Part model, mm, in its own coordinate system. Round coordinates to 2 decimals unless told otherwise and drop trailing zeros. Write each loop counter-clockwise with the first axis right and the second up, starting at its lowest first coordinate (ties: lowest second). Pieces come first, ordered by that corner, then holes. Notation, with made-up numbers: M 54,86 L 99,86 A7 ccw 99,96 Z; hole C 59.25,-21 d1. An arc over 180 degrees is marked long. Use a Markdown table: item, result. Add a question column.
1) Slice it at C-C on z = -3. Write the cut outline in (x, y).
2) Slice it at B-B on x = 20. Write the cut outline in (y, z), plus the area to 3 significant figures.
3) Drop flat-ended pins along their axis: P1, Ø1, axis at x = -9.5, z = -1, coming from the -Y side; P2, Ø5, axis at x = -29.5, z = 3.5, coming from the -Y side; P3, Ø3, axis at x = 31.5, y = 0, coming from the -Z side. Give the stop position or say it passes through.
4) Wall check: probe 1 along Y at (x, z) = (-17, 0); probe 2 along X at (y, z) = (4, -1); probe 3 along X at (y, z) = (1.5, -3.25). Give the ranges that are in metal, low to high.
5) Slice it at A-A on y = 0. Write the cut outline in (x, z).
```python
from build123d import *

# Parameters (mm, degrees)
SKETCH1_R      = 1.27
EXTRUDE1_DEPTH = 44.45


with BuildPart() as part:
    # Sketch1 → Extrude1 (new, symmetric)
    with BuildSketch(Plane(origin=(0, 0, 0), x_dir=(0, 0, -1), z_dir=(1, 0, 0))):
        Circle(SKETCH1_R)
    extrude(amount=EXTRUDE1_DEPTH, both=True)

    # Sketch2 → Revolve1 (revolve)
    with BuildSketch(Plane.ZY.offset(44.45)):
        with BuildLine():
            Line((0, -5.1054), (0, 5.1054))
            ThreePointArc((0, 5.1054), (-5.1054, 0), (0, -5.1054))
        make_face()
    revolve(axis=Axis((-44.45, 8.762723072, 0), (0, -1, 0)))

    # Sketch3 → Revolve2 (revolve)
    with BuildSketch(Plane(origin=(44.45, 0, 0), x_dir=(0, 0, -1), z_dir=(1, 0, 0))):
        with BuildLine():
            Line((0, 5.1054), (0, -5.1054))
            ThreePointArc((0, -5.1054), (5.1054, 0), (0, 5.1054))
        make_face()
    revolve(axis=Axis((44.45, 5.1054, 0), (0, -1, 0)))


solid = part.part
```
Entries:
| question | item | result |
|---|---|---|
| 1 | outline | C -44.45,0 d8.26; C 44.45,0 d8.26 |
| 2 | outline | C 0,0 d2.54 |
| 2 | area | 5.07 mm^2 |
| 3 | P1 | stops at y = -1.17 |
| 3 | P2 | stops at y = -0.78 |
| 3 | P3 | stops at z = -1.27 |
| 4 | probe 1 | y = -1.27 to 1.27 |
| 4 | probe 2 | x = -47.46 to -41.44, 41.44 to 47.46 |
| 4 | probe 3 | x = -48.09 to -40.81, 40.81 to 48.09 |
| 5 | outline | M -39.51,-1.27 L 39.51,-1.27 A5.11 ccw long 39.51,1.27 L -39.51,1.27 A5.11 ccw long Z |
